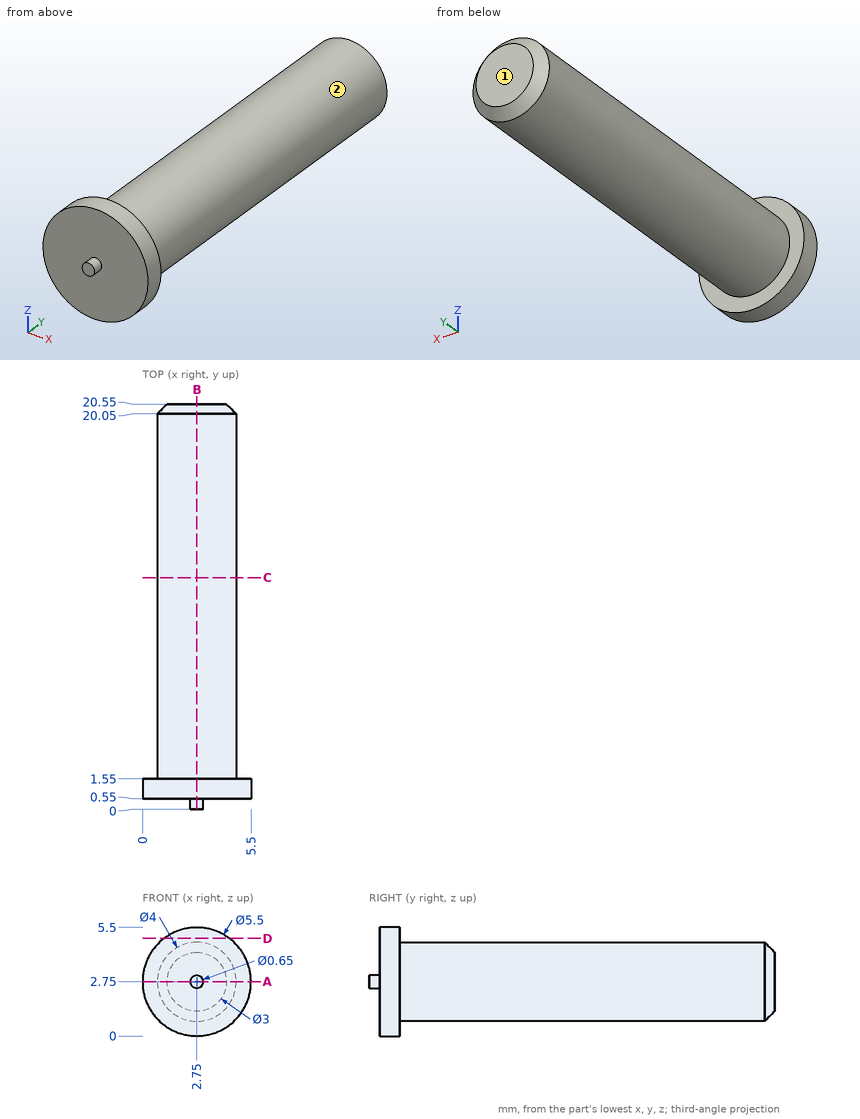
Drawing for the job (mm, zero at the part's lowest x, y, z). A direction names the side the tool comes from. Round coordinates to 2 decimals unless told otherwise and drop trailing zeros. Loops run counter-clockwise (first coordinate to the right, second up) from the corner with the lowest first, then second, coordinate; pieces in that order, holes last. Notation, with made-up numbers: M 36.5,73 L 79.5,73 A13 ccw 79.5,95 Z; hole C 66,-14.5 d9. An arc over 180 degrees is marked long. Use a Markdown table: item, result. Add a question column.
(1) Cut at C-C (y = 11.75). Give the cut face in (x, z).
(2) Cut at A-A (z = 2.75). Give the cut face in (x, y) (3 decimals), and give its area (3 significant figures).
(3) Cut at D-D (z = 4.95). Give the cut face in (x, y).
(4) Drill centre lines: line 1 (Y direction, x = 3.7, z = 3.5); line 2 (Y direction, x = 4.75, z = 3.9); line 3 (X direction, y = 4, z = 2.7). Where is each one in solid material? Low to high.
(5) Flat gauge pin, fed straight in: pin 1 (3 mm diameter, centred on x = 2, y = 7, fed in from -Z). Where does the tip first touch, or does it go through?
(6) Which spindle directions (+Z, -Z, +X, -X, +Y, -Y) get a long thin tool onto all of the face, cutting with end or side? Do the marked faces 1 and 2. Say none if no direction does.
(7) Cut at B-B (x = 2.75). Give the cut face in (y, z) (3 decimals), and give its area (3 significant figures).
Geometry says:
| question | item | result |
|---|---|---|
| 1 | outline | C 2.75,2.75 d4 |
| 2 | outline | M 0,0.55 L 2.425,0.55 L 2.425,0 L 3.075,0 L 3.075,0.55 L 5.5,0.55 L 5.5,1.55 L 4.75,1.55 L 4.75,20.05 L 4.25,20.55 L 1.25,20.55 L 0.75,20.05 L 0.75,1.55 L 0,1.55 Z |
| 2 | area | 81.6 mm² |
| 3 | outline | M 1.1,0.55 L 4.4,0.55 L 4.4,1.55 L 1.1,1.55 Z |
| 4 | line 1 | y = 0.55 to 20.55 |
| 4 | line 2 | y = 0.55 to 1.55 |
| 4 | line 3 | x = 0.75 to 4.75 |
| 5 | pin 1 | stops at z = 0.75 |
| 6 | face 1 | +Z, -Z, +X, -X, +Y |
| 6 | face 2 | +Y |
| 7 | outline | M 0,2.425 L 0.55,2.425 L 0.55,0 L 1.55,0 L 1.55,0.75 L 20.05,0.75 L 20.55,1.25 L 20.55,4.25 L 20.05,4.75 L 1.55,4.75 L 1.55,5.5 L 0.55,5.5 L 0.55,3.075 L 0,3.075 Z |
| 7 | area | 81.6 mm² |
